Geometry: final body of the model. Coordinates: model frame, mm. A direction names the side the tool comes from. Round coordinates to 2 decimals unless told otherwise and drop trailing zeros. Loops run counter-clockwise (first coordinate to the right, second up) from the corner with the lowest first, then second, coordinate; pieces in that order, holes last. Notation, with made-up numbers: (6, -1.5) - (24, -1.5) arc R26 ccw to (24, 31.5) - close; hole circle Ø8 at (64.5, 88). An arc over 180 degrees is marked (long way). Answer in a Markdown table with one row per item. Add a question column.
from build123d import *

# Parameters (mm, degrees)
SKETCH1_R           = 15
BOSS_EXTRUDE1_DEPTH = 54
BOSS_EXTRUDE2_DEPTH = 10
SKETCH4_W           = 12.7
SKETCH4_H           = 25
CUT_EXTRUDE2_DEPTH  = 12.7
CHAMFER1_SIZE       = 1
CHAMFER1_SIZE2      = 0.707106781
SKETCH6_R           = 2.6
CUT_EXTRUDE3_DEPTH  = 93.478960977
SKETCH7_R           = 1.8
BOSS_EXTRUDE4_DEPTH = 5
FILLET1_R           = 5
SKETCH8_W           = 60
SKETCH8_H           = 60
BOSS_EXTRUDE5_DEPTH = 10
BOSS_EXTRUDE6_DEPTH = 4
FILLET2_R           = 5
SKETCH10_R          = 5
CUT_EXTRUDE4_DEPTH  = 104.462384491
CHAMFER2_SIZE       = 8
EXTRUDE_THIN1_START = 2
SKETCH11_R          = 3.4
SKETCH11_R_2        = 1.8
EXTRUDE_THIN1_DEPTH = 2
SKETCH12_W          = 50
SKETCH12_H          = 14
CUT_EXTRUDE5_DEPTH  = 2
CHAMFER3_SIZE       = 2
CUT_EXTRUDE6_DEPTH  = 2
SKETCH14_R          = 8
CUT_EXTRUDE7_DEPTH  = 44
CHAMFER4_SIZE       = 3
CUT_EXTRUDE8_DEPTH  = 104.462384491
SKETCH26_R          = 2.5
CUT_EXTRUDE16_DEPTH = 37
CUT_EXTRUDE17_DEPTH = 9
CHAMFER6_SIZE       = 3
SKETCH29_W          = 1.35
SKETCH29_H          = 25
CUT_EXTRUDE18_DEPTH = 12.7


# Some blends are built 0.0001 mm under size
with BuildPart() as part:
    # Sketch1 → Boss-Extrude1 (new body)
    with BuildSketch(Plane(origin=(0, 0, 0), x_dir=(1, 0, 0), z_dir=(0, 1, 0))):
        with Locations(Location((0, 0, 0), (0, 0, 270))):
            Circle(SKETCH1_R)
    extrude(amount=BOSS_EXTRUDE1_DEPTH)

    # Sketch2 → Boss-Extrude2 (add, symmetric)
    with BuildSketch(Plane(origin=(0, 0, 0), x_dir=(0, 0, -1), z_dir=(1, 0, 0))):
        Polygon((-15, 54), (20.355339059, 54), (20.355339059, 69), (2.67766953, 86.67766953), (-15, 69), align=None)
    extrude(amount=BOSS_EXTRUDE2_DEPTH, both=True)

    # Sketch4 → Cut-Extrude2 (cut)
    with BuildSketch(Plane(origin=(0, 42, 42), x_dir=(1, 0, 0), z_dir=(0, 0.7071067811865467, 0.7071067811865485))):
        with Locations((-6.35, 50.683766184)):
            Rectangle(SKETCH4_W, SKETCH4_H)
    extrude(amount=-CUT_EXTRUDE2_DEPTH, mode=Mode.SUBTRACT)

    # Chamfer1
    chamfer1_edges = [part.edges().sort_by_distance(p)[0] for p in [
        (-5, 69, 15),
    ]]
    chamfer1_side = [part.faces().sort_by_distance(p)[0] for p in [
        (0, 61.5, 15),
    ]]
    chamfer(chamfer1_edges, length=CHAMFER1_SIZE, length2=CHAMFER1_SIZE2, reference=chamfer1_side[0])

    # Sketch6 → Cut-Extrude3 (cut, through all)
    with BuildSketch(Plane(origin=(10, 0, 0), x_dir=(0, 0, -1), z_dir=(1, 0, 0))):
        with Locations((3.632263684, 78.652007563)):
            Circle(SKETCH6_R)
        with Locations((-6.974338034, 68.045405845)):
            Circle(SKETCH6_R)
    extrude(amount=-CUT_EXTRUDE3_DEPTH, mode=Mode.SUBTRACT)

    # Sketch7 → Boss-Extrude4 (add)
    with BuildSketch(Plane.XY.offset(15)):
        with BuildLine():
            Line((-31, 0), (31, 0))
            ThreePointArc((31, 0), (33.828427125, 1.171572875), (35, 4))
            Line((35, 4), (35, 50))
            ThreePointArc((35, 50), (33.828427125, 52.828427125), (31, 54))
            Line((31, 54), (-31, 54))
            ThreePointArc((-31, 54), (-33.828427125, 52.828427125), (-35, 50))
            Line((-35, 50), (-35, 4))
            ThreePointArc((-35, 4), (-33.828427125, 1.171572875), (-31, 0))
        make_face()
        with Locations((-30, 49)):
            Circle(SKETCH7_R, mode=Mode.SUBTRACT)
        with Locations((30, 49)):
            Circle(SKETCH7_R, mode=Mode.SUBTRACT)
        with Locations((30, 5)):
            Circle(SKETCH7_R, mode=Mode.SUBTRACT)
        with Locations((-30, 5)):
            Circle(SKETCH7_R, mode=Mode.SUBTRACT)
    extrude(amount=-BOSS_EXTRUDE4_DEPTH)

    # Fillet1
    fillet1_edges = [part.edges().sort_by_distance(p)[0] for p in [
        (11.180339887, 27, 10),
        (-11.180339887, 27, 10),
    ]]
    fillet(fillet1_edges, radius=FILLET1_R)

    # Sketch8 → Boss-Extrude5 (add)
    with BuildSketch(Plane.XZ):
        with Locations((0, -30)):
            Rectangle(SKETCH8_W, SKETCH8_H)
    extrude(amount=-BOSS_EXTRUDE5_DEPTH)

    # Sketch9 → Boss-Extrude6 (add, symmetric)
    with BuildSketch(Plane(origin=(0, 0, 0), x_dir=(0, 0, -1), z_dir=(1, 0, 0))):
        Polygon((15, 50), (55, 10), (10, 10), (10, 50), align=None)
    extrude(amount=BOSS_EXTRUDE6_DEPTH, both=True)

    # Fillet2
    fillet2_edges = [part.edges().sort_by_distance(p)[0] for p in [
        (-30, 5, 0),
        (30, 5, 0),
        (30, 5, -60),
        (-30, 5, -60),
    ]]
    fillet(fillet2_edges, radius=FILLET2_R)

    # Sketch10 → Cut-Extrude4 (cut, through all)
    with BuildSketch(Plane(origin=(0, 10, 0), x_dir=(1, 0, 0), z_dir=(0, 1, 0))):
        with Locations(Location((15, 45, 0), (0, 0, 270))):
            Circle(SKETCH10_R)
        with Locations(Location((-15, 45, 0), (0, 0, 270))):
            Circle(SKETCH10_R)
        with Locations(Location((-15, 15, 0), (0, 0, 270))):
            Circle(SKETCH10_R)
        with Locations(Location((15, 15, 0), (0, 0, 270))):
            Circle(SKETCH10_R)
    extrude(amount=-CUT_EXTRUDE4_DEPTH, mode=Mode.SUBTRACT)

    # Chamfer2
    # the kernel refuses this chamfer: 8 mm, written as the material it takes off along each edge
    with BuildSketch(Plane(origin=(-30.573463904, 54, -20.355339059), x_dir=(0, -0.027495876610586487, 0.9996219169112968), z_dir=(1, 0, 0))) as chamfer2_piece_1_section:
        Polygon((CHAMFER2_SIZE * 0.999621916911, -CHAMFER2_SIZE * 0.0274958766106), (-CHAMFER2_SIZE * 0.0274958766106, -CHAMFER2_SIZE * 0.999621916911), (0, 0), align=None)
    chamfer2_piece_1 = extrude(amount=61.146927807, mode=Mode.PRIVATE)
    chamfer2_piece_1 = chamfer2_piece_1 - Plane(origin=(0, 56.680646847, 0), x_dir=(0, 0, 1), z_dir=(0, -1, 0)) * Cylinder(15, 155, mode=Mode.PRIVATE)
    add(chamfer2_piece_1, mode=Mode.SUBTRACT)

    # Sketch11 → Extrude-Thin1 (add)
    # profile 1 of 4: a face of its own
    with BuildSketch(Plane.XY.offset(15).offset(EXTRUDE_THIN1_START)):
        with Locations((-30, 49)):
            Circle(SKETCH11_R)
        with Locations((-30, 49)):
            Circle(SKETCH11_R_2, mode=Mode.SUBTRACT)
    # profile 2 of 4: a face of its own
    with BuildSketch(Plane.XY.offset(15).offset(EXTRUDE_THIN1_START)):
        with Locations((30, 49)):
            Circle(SKETCH11_R)
        with Locations((30, 49)):
            Circle(SKETCH11_R_2, mode=Mode.SUBTRACT)
    # profile 3 of 4: a face of its own
    with BuildSketch(Plane.XY.offset(15).offset(EXTRUDE_THIN1_START)):
        with Locations((30, 5)):
            Circle(SKETCH11_R)
        with Locations((30, 5)):
            Circle(SKETCH11_R_2, mode=Mode.SUBTRACT)
    # profile 4 of 4: a face of its own
    with BuildSketch(Plane.XY.offset(15).offset(EXTRUDE_THIN1_START)):
        with Locations((-30, 5)):
            Circle(SKETCH11_R)
        with Locations((-30, 5)):
            Circle(SKETCH11_R_2, mode=Mode.SUBTRACT)
    extrude(amount=-EXTRUDE_THIN1_DEPTH)

    # Sketch12 → Cut-Extrude5 (cut)
    with BuildSketch(Plane.XY.offset(15)):
        with Locations((0, 52)):
            Rectangle(SKETCH12_W, SKETCH12_H)
    extrude(amount=-CUT_EXTRUDE5_DEPTH, mode=Mode.SUBTRACT)

    # Chamfer3
    chamfer3_edges = [part.edges().sort_by_distance(p)[0] for p in [
        (0, 59, 13),
    ]]
    chamfer(chamfer3_edges, length=CHAMFER3_SIZE - 0.0001)  # a hair under: the kernel refuses the full size

    # Sketch13 → Cut-Extrude6 (cut)
    with BuildSketch(Plane(origin=(0, 0, 10), x_dir=(-1, 0, 0), z_dir=(0, 0, -1))):
        Polygon((-30, 45.882308546), (-27.3, 47.441154273), (-27.3, 50.558845727), (-30, 52.117691454), (-32.7, 50.558845727), (-32.7, 47.441154273), align=None)
        Polygon((30, 45.882308546), (32.7, 47.441154273), (32.7, 50.558845727), (30, 52.117691454), (27.3, 50.558845727), (27.3, 47.441154273), align=None)
        Polygon((27.3, 6.558845727), (27.3, 3.441154273), (30, 1.882308546), (32.7, 3.441154273), (32.7, 6.558845727), (30, 8.117691454), align=None)
        Polygon((-32.7, 6.558845727), (-32.7, 3.441154273), (-30, 1.882308546), (-27.3, 3.441154273), (-27.3, 6.558845727), (-30, 8.117691454), align=None)
    extrude(amount=-CUT_EXTRUDE6_DEPTH, mode=Mode.SUBTRACT)

    # Sketch14 → Cut-Extrude7 (cut)
    with BuildSketch(Plane(origin=(0, 10, 0), x_dir=(1, 0, 0), z_dir=(0, 1, 0))):
        with Locations((15, 15)):
            Circle(SKETCH14_R)
        with Locations((-15, 15)):
            Circle(SKETCH14_R)
    extrude(amount=CUT_EXTRUDE7_DEPTH, mode=Mode.SUBTRACT)

    # Chamfer4
    chamfer4_edges = [part.edges().sort_by_distance(p)[0] for p in [
        (15, 10, -20),
        (-15, 10, -20),
        (-15, 10, -50),
        (15, 10, -50),
    ]]
    chamfer(chamfer4_edges, length=CHAMFER4_SIZE - 0.0001)  # a hair under: the kernel refuses the full size

    # Sketch15 → Cut-Extrude8 (cut, through all)
    with BuildSketch(Plane(origin=(0, 10, 0), x_dir=(1, 0, 0), z_dir=(0, 1, 0))):
        with BuildLine():
            Line((4, 22), (4, 38))
            ThreePointArc((4, 38), (12, 30), (4, 22))
        make_face()
    extrude(amount=-CUT_EXTRUDE8_DEPTH, mode=Mode.SUBTRACT)

    # Sketch26 → Cut-Extrude16 (cut)
    with BuildSketch(Plane(origin=(0, 33.019743879, 33.019743879), x_dir=(1, 0, 0), z_dir=(0, 0.7071067811865466, 0.7071067811865485))):
        with Locations(Location((-5, 58.183766184, 0), (0, 0, 270))):
            Circle(SKETCH26_R)
        with Locations(Location((-5, 43.183766184, 0), (0, 0, 270))):
            Circle(SKETCH26_R)
    extrude(amount=-CUT_EXTRUDE16_DEPTH, mode=Mode.SUBTRACT)

    # Sketch27 → Cut-Extrude17 (cut)
    with BuildSketch(Plane.ZY.offset(10)):
        Polygon((-20.355339059, 62), (-6.17766953, 47.82233047), (-27.390872965, 26.609127035), (-41.568542495, 40.786796564), align=None)
    extrude(amount=-CUT_EXTRUDE17_DEPTH, mode=Mode.SUBTRACT)

    # Chamfer6
    chamfer6_edges = [part.edges().sort_by_distance(p)[0] for p in [
        (-4, 29.359127035, -30.140872965),
    ]]
    chamfer(chamfer6_edges, length=CHAMFER6_SIZE - 0.0001)  # a hair under: the kernel refuses the full size

    # Sketch29 → Cut-Extrude18 (cut)
    with BuildSketch(Plane(origin=(0, 42, 42), x_dir=(1, 0, 0), z_dir=(0, 0.7071067811865461, 0.7071067811865489))):
        with Locations((0.675, 50.683766184)):
            Rectangle(SKETCH29_W, SKETCH29_H)
    extrude(amount=-CUT_EXTRUDE18_DEPTH, mode=Mode.SUBTRACT)


solid = part.part
1) Reachability of faces 4 (the flat face through (0, 65, -20.355)), 5 (the flat face through (27, 27, 10)), 6 (the flat face through (-2.479, 28.275, -31.148)) from +Z, -Z, +X, -X, +Y, -Y: full face, straight path, thin tool, end or side. Return the list, or none.
2) Pull-direction query (Y, two-part tool) for faces 1 (the cylindrical face through (29, 5, -58)), 2 (the cylindrical face through (-33.859, 1.203, 12.535)), 3 (the flat face through (-10, 48, -8)); classes: pulls with the +Y half, pulls with the -Y half, needs draft (parallel to the pull), parting line crosses it, or undercut.
3) Section A-A, the plane z = -45. Return the cut outline in (x, y).
4) Section D-D, the plane y = 23. Return the cut outline in (x, z).
5) Section B-B, the plane y = 11.5. Return the cut outline in (x, z).
6) Contact query for flat-ended pins moving along their axis: pin 1 Ø5 at (y, z) = (4.5, -29) entering from +X; pin 2 Ø13.5 at (y, z) = (76.5, 6.5) entering from -X; pin 3 Ø12 at (x, y) = (-13.5, 34.5) entering from +Z. Output: stop coordinate, or through.
7) Material intervals for line 1 along Y through (x, z) = (30, 14.1); line 2 along X through (y, z) = (3, -45); line 3 along Z through (x, y) = (20.5, 46), sorted ascending. Write a range as from..to.
Evaluation:
| question | item | result |
|---|---|---|
| 1 | face 4 | -Z, +X, -X, +Y |
| 1 | face 5 | +X, +Y, -Y |
| 1 | face 6 | -X, +Y |
| 2 | face 1 | needs draft |
| 2 | face 2 | pulls with the -Y half |
| 2 | face 3 | undercut |
| 3 | outline | (-30, 0) - (-20, 0) - (-20, 7) - (-23, 10) - (-30, 10) - close; (-10, 0) - (10, 0) - (10, 7) - (7, 10) - (4, 10) - (4, 20) - (-4, 20) - (-4, 10) - (-7, 10) - (-10, 7) - close; (20, 0) - (30, 0) - (30, 10) - (23, 10) - (20, 7) - close |
| 4 | outline | (-35, 10) - (-19.36, 10) arc R5 cw to (-14.52, 3.75) arc R15 ccw to (-13.15, -7.22) arc R8 cw to (-7.22, -13.15) arc R15 ccw to (-4, -14.46) - (-4, -42) - (4, -42) - (4, -14.46) arc R15 ccw to (7.22, -13.15) arc R8 cw to (13.15, -7.22) arc R15 ccw to (14.52, 3.75) arc R5 cw to (19.36, 10) - (35, 10) - (35, 15) - (-35, 15) - close |
| 5 | outline | (-35, 10) - (-19.36, 10) arc R5 cw to (-14.52, 3.75) arc R15 ccw to (-13.15, -7.22) arc R8 cw to (-7.22, -13.15) arc R15 ccw to (-4, -14.46) - (-4, -53.5) - (4, -53.5) - (4, -14.46) arc R15 ccw to (7.22, -13.15) arc R8 cw to (13.15, -7.22) arc R15 ccw to (14.52, 3.75) arc R5 cw to (19.36, 10) - (35, 10) - (35, 15) - (-35, 15) - close |
| 6 | pin 1 | stops at x = 30 |
| 6 | pin 2 | stops at x = 1.35 |
| 6 | pin 3 | stops at z = 15 |
| 7 | line 1 | y = 0..3.2, 6.8..47.2, 50.8..54 |
| 7 | line 2 | x = -30..-20, -10..10, 20..30 |
| 7 | line 3 | z = 10..13 |
